Geometry: final body of the model. Coordinates: model frame, mm. A direction names the side the tool comes from. Round coordinates to 2 decimals unless told otherwise and drop trailing zeros. Order: outer loops, then holes, each group sorted by start corner. A loop starts at its lowest first (then second) coordinate and runs counter-clockwise, first axis right, second up. Notation, with made-up numbers: M 73,-15.75 L 111,-15.75 A9 ccw 111,1.25 Z; hole C -24,13 d10. An arc over 180 degrees is marked long. Return JSON: item names as keys, results as strings. Group by question number.
Q1. Cut plane B-B on x = -70. Output: boundary loops of the cut face in (y, z).
Q2. Cut plane D-D on y = 140.5. Output: boundary loops of the cut face in (x, z).
Q3. Cut plane A-A on z = 14. Count the separate pieces of the cut face and the enclosed holes in it, and give its area (3 significant figures).
Q4. Mould query, pull axis Y, two halves, no side actions, for faces 1 (the face through (20, 185, 11)), 2 (the face through (-13, 125.374, 4)), 3 (the face through (19, 132, 5)). Classes: released by +Y, released by -Y, zero draft, split by the parting line, or undercut.
Q5. Ray query, probe 1 along Y at (x, z) = (-129.5, 12); probe 2 along Y at (x, z) = (-156, 8.5); probe 3 along Y at (x, z) = (-104, 3). Return the intervals inside material, ascending.
Q6. Access query for faces 4 (the face through (3, 273.974, 3)), 5 (the face through (-50, 173, 11)), 6 (the face through (33.2, 253.5, 21.3)), 7 (the face through (-129, 156, 5)). Directions: +Z, -Z, +X, -X, +Y, -Y. A direction counts if a zero-diameter tool reaches every point of the face in a straight line with its end or side. Return the directions, or none.
Q7. Cut plane C-C on z = 27.5. Output: boundary loops of the cut face in (x, y) (3 decimals).
Q8. Contact query for flat-ended pins moving along their axis: pin 1 (13 mm diameter, centred on x = -132, y = 152, fed in from +Z); pin 2 (7.5 mm diameter, centred on x = -59.5, z = 11.5, fed in from +Y); pin 3 (4 mm diameter, centred on x = -161.5, z = 3, fed in from -Y); pin 4 (12 mm diameter, centred on x = 50.5, z = 24, fed in from +Y). Output: stop coordinate, or through.
```python
from build123d import *

# Parameters (mm, degrees)
SKETCH1_W            = 128
SKETCH1_H            = 110
SKETCH1_W_2          = 50
SKETCH1_H_2          = 70
BOSS_EXTRUDE1_DEPTH  = 5
SKETCH2_R            = 4.5
SKETCH2_R_2          = 3.025
SKETCH2_R_3          = 4.411768353
BOSS_EXTRUDE2_DEPTH  = 6
SKETCH3_W            = 194
SKETCH3_H            = 2
BOSS_EXTRUDE3_DEPTH  = 20
SKETCH6_W            = 12
SKETCH6_H            = 12
BOSS_EXTRUDE5_DEPTH  = 5
M4_CLEARANCE_HOLE1_D = 4.8
CUT_EXTRUDE1_DEPTH   = 329.83563266
FILLET2_R            = 3
FILLET3_R            = 3
SKETCH11_R           = 5
SKETCH11_R_2         = 3.025
BOSS_EXTRUDE6_DEPTH  = 30
FILLET4_R            = 3


with BuildPart() as part:
    # Sketch1 → Boss-Extrude1 (new body)
    with BuildSketch(Plane.XY):
        with Locations((-103.32475602, 215.37439567)):
            Rectangle(SKETCH1_W, SKETCH1_H)
        Polygon((26.67524398, 270.37439567), (-39.32475602, 270.37439567), (-39.32475602, 160.37439567), (-39.32475602, 125.37439567), (26.67524398, 125.37439567), (26.67524398, 195.37439567), (26.67524398, 200.37439567), align=None)
        with Locations((51.67524398, 235.37439567)):
            Rectangle(SKETCH1_W_2, SKETCH1_H_2)
    extrude(amount=BOSS_EXTRUDE1_DEPTH)

    # Sketch2 → Boss-Extrude2 (add)
    # profile 1 of 10: a face of its own
    with BuildSketch(Plane.XY.offset(5)):
        with Locations((-49.57975602, 169.52739567)):
            Circle(SKETCH2_R)
        with Locations((-49.57975602, 169.52739567)):
            Circle(SKETCH2_R_2, mode=Mode.SUBTRACT)
    # profile 2 of 10: a face of its own
    with BuildSketch(Plane.XY.offset(5)):
        with Locations((-31.18175602, 188.30539567)):
            Circle(SKETCH2_R)
        with Locations((-31.18175602, 188.30539567)):
            Circle(SKETCH2_R_2, mode=Mode.SUBTRACT)
    # profile 3 of 10: a face of its own
    with BuildSketch(Plane.XY.offset(5)):
        with Locations((-31.18175602, 131.55539567)):
            Circle(SKETCH2_R)
        with Locations((-31.18175602, 131.55539567)):
            Circle(SKETCH2_R_2, mode=Mode.SUBTRACT)
    # profile 4 of 10: a face of its own
    with BuildSketch(Plane.XY.offset(5)):
        with Locations((18.81824398, 131.55539567)):
            Circle(SKETCH2_R)
        with Locations((18.81824398, 131.55539567)):
            Circle(SKETCH2_R_2, mode=Mode.SUBTRACT)
    # profile 5 of 10: a face of its own
    with BuildSketch(Plane.XY.offset(5)):
        with Locations((18.81824398, 188.30539567)):
            Circle(SKETCH2_R)
        with Locations((18.81824398, 188.30539567)):
            Circle(SKETCH2_R_2, mode=Mode.SUBTRACT)
    # profile 6 of 10: a face of its own
    with BuildSketch(Plane.XY.offset(5)):
        with Locations((18.81824398, 261.55539567)):
            Circle(SKETCH2_R)
        with Locations((18.81824398, 261.55539567)):
            Circle(SKETCH2_R_2, mode=Mode.SUBTRACT)
    # profile 7 of 10: a face of its own
    with BuildSketch(Plane.XY.offset(5)):
        with Locations((-49.57975602, 262.49139567)):
            Circle(SKETCH2_R_3)
        with Locations((-49.57975602, 262.49139567)):
            Circle(SKETCH2_R_2, mode=Mode.SUBTRACT)
    # profile 8 of 10: a face of its own
    with BuildSketch(Plane.XY.offset(5)):
        with Locations((-154.35475602, 262.49139567)):
            Circle(SKETCH2_R)
        with Locations((-154.35475602, 262.49139567)):
            Circle(SKETCH2_R_2, mode=Mode.SUBTRACT)
    # profile 9 of 10: a face of its own
    with BuildSketch(Plane.XY.offset(5)):
        with Locations((-154.35475602, 169.52739567)):
            Circle(SKETCH2_R)
        with Locations((-154.35475602, 169.52739567)):
            Circle(SKETCH2_R_2, mode=Mode.SUBTRACT)
    # profile 10 of 10: a face of its own
    with BuildSketch(Plane.XY.offset(5)):
        with Locations((-31.18175602, 261.55539567)):
            Circle(SKETCH2_R)
        with Locations((-31.18175602, 261.55539567)):
            Circle(SKETCH2_R_2, mode=Mode.SUBTRACT)
    extrude(amount=BOSS_EXTRUDE2_DEPTH)

    # Sketch3 → Boss-Extrude3 (add)
    with BuildSketch(Plane.XY.offset(5)):
        with Locations((-70.32475602, 269.37439567)):
            Rectangle(SKETCH3_W, SKETCH3_H)
        Polygon((-167.32475602, 162.37439567), (-167.32475602, 160.37439567), (-39.32475602, 160.37439567), (-39.32475602, 125.37439567), (-37.32475602, 125.37439567), (-37.32475602, 162.37439567), align=None)
    extrude(amount=BOSS_EXTRUDE3_DEPTH)

    # Sketch6 → Boss-Extrude5 (add)
    with BuildSketch(Plane(origin=(0, 0, 0), x_dir=(-1, 0, 0), z_dir=(0, 0, -1))):
        with Locations((131.32475602, 154.37439567)):
            Rectangle(SKETCH6_W, SKETCH6_H)
        with Locations((159.32475602, 276.37439567)):
            Rectangle(SKETCH6_W, SKETCH6_H)
        with Locations((45.32475602, 154.37439567)):
            Rectangle(SKETCH6_W, SKETCH6_H)
        with Locations((-5.67524398, 276.37439567)):
            Rectangle(SKETCH6_W, SKETCH6_H)
    extrude(amount=-BOSS_EXTRUDE5_DEPTH)

    # M4 Clearance Hole1 (through all)
    with Locations(Plane.XY.offset(5)):
        with Locations((-131.32475602, 154.37439567), (-159.32475602, 276.37439567), (5.67524398, 276.37439567), (-45.32475602, 154.37439567)):
            Hole(M4_CLEARANCE_HOLE1_D / 2)

    # Sketch10 → Cut-Extrude1 (cut, through all)
    with BuildSketch(Plane.XY.offset(5)):
        with BuildLine():
            ThreePointArc((-131.32475602, 151.97439567), (-133.72475602, 154.37439567), (-131.32475602, 156.77439567))
            Line((-131.32475602, 156.77439567), (-137.32475602, 156.77439567))
            Line((-137.32475602, 156.77439567), (-137.32475602, 151.97439567))
            Line((-137.32475602, 151.97439567), (-131.32475602, 151.97439567))
        make_face()
        with BuildLine():
            ThreePointArc((-159.32475602, 273.97439567), (-161.72475602, 276.37439567), (-159.32475602, 278.77439567))
            Line((-159.32475602, 278.77439567), (-165.32475602, 278.77439567))
            Line((-165.32475602, 278.77439567), (-165.32475602, 273.97439567))
            Line((-165.32475602, 273.97439567), (-159.32475602, 273.97439567))
        make_face()
        with BuildLine():
            ThreePointArc((5.67524398, 273.97439567), (3.27524398, 276.37439567), (5.67524398, 278.77439567))
            Line((5.67524398, 278.77439567), (-0.32475602, 278.77439567))
            Line((-0.32475602, 278.77439567), (-0.32475602, 273.97439567))
            Line((-0.32475602, 273.97439567), (5.67524398, 273.97439567))
        make_face()
        with BuildLine():
            ThreePointArc((-45.32475602, 151.97439567), (-47.72475602, 154.37439567), (-45.32475602, 156.77439567))
            Line((-45.32475602, 156.77439567), (-51.32475602, 156.77439567))
            Line((-51.32475602, 156.77439567), (-51.32475602, 151.97439567))
            Line((-51.32475602, 151.97439567), (-45.32475602, 151.97439567))
        make_face()
    extrude(amount=-CUT_EXTRUDE1_DEPTH, mode=Mode.SUBTRACT)

    # Fillet2
    # the kernel refuses this fillet: 3 mm, written as the material it adds along each edge
    with BuildSketch(Plane(origin=(-137.32475602, 160.37439567, 0), x_dir=(-1, 0, 0), z_dir=(0, 0, 1)), Plane(origin=(-153.32475602, 270.37439567, 0), x_dir=(1, 0, 0), z_dir=(0, 0, 1)), Plane(origin=(-51.32475602, 160.37439567, 0), x_dir=(-1, 0, 0), z_dir=(0, 0, 1)), Plane(origin=(11.67524398, 270.37439567, 0), x_dir=(1, 0, 0), z_dir=(0, 0, 1))) as fillet2_piece_1:
        with BuildLine():
            CenterArc((FILLET2_R, FILLET2_R), FILLET2_R, 180, 90)
            Line((0, FILLET2_R), (0, 0))
            Line((0, 0), (FILLET2_R, 0))
        make_face()
    extrude(amount=5)
    with BuildSketch(Plane(origin=(-125.32475602, 160.37439567, 0), x_dir=(1, 0, 0), z_dir=(0, 0, 1)), Plane(origin=(-39.32475602, 148.37439567, 0), x_dir=(0, -1, 0), z_dir=(0, 0, 1)), Plane(origin=(-0.32475602, 270.37439567, 0), x_dir=(-1, 0, 0), z_dir=(0, 0, 1))) as fillet2_piece_2:
        with BuildLine():
            CenterArc((FILLET2_R, -FILLET2_R), FILLET2_R, 90, 90)
            Line((0, -FILLET2_R), (0, 0))
            Line((0, 0), (FILLET2_R, 0))
        make_face()
    extrude(amount=5)
    with BuildSketch(Plane(origin=(-165.32475602, 270.37439567, 0), x_dir=(-1, 0, 0), z_dir=(0, 0, 1))) as fillet2_piece_3:
        with BuildLine():
            CenterArc((3, -2.828427125), FILLET2_R, 109.471220634, 70.528779366)
            Line((0, -2.828427125), (0, 0))
            Line((0, 0), (2, 0))
        make_face()
    extrude(amount=5)
    # the kernel refuses this fillet: 3 mm, written as the material it takes off along each edge
    with BuildSketch(Plane(origin=(-125.32475602, 148.37439567, -7.5), x_dir=(0, 1, 0), z_dir=(0, 0, 1))) as fillet2_2_piece_1:
        with BuildLine():
            CenterArc((FILLET2_R, FILLET2_R), FILLET2_R, 180, 90)
            Line((0, FILLET2_R), (0, 0))
            Line((0, 0), (FILLET2_R, 0))
        make_face()
    extrude(amount=20, mode=Mode.SUBTRACT)
    with BuildSketch(Plane(origin=(-153.32475602, 282.37439567, -7.5), x_dir=(0, -1, 0), z_dir=(0, 0, 1)), Plane(origin=(11.67524398, 282.37439567, -7.5), x_dir=(0, -1, 0), z_dir=(0, 0, 1))) as fillet2_2_piece_2:
        with BuildLine():
            CenterArc((FILLET2_R, -FILLET2_R), FILLET2_R, 90, 90)
            Line((0, -FILLET2_R), (0, 0))
            Line((0, 0), (FILLET2_R, 0))
        make_face()
    extrude(amount=20, mode=Mode.SUBTRACT)

    # Fillet3
    fillet3_edges = [part.edges().sort_by_distance(p)[0] for p in [
        (76.67524398, 270.37439567, 2.5),
        (76.67524398, 200.37439567, 2.5),
        (26.67524398, 200.37439567, 2.5),
        (26.67524398, 125.37439567, 2.5),
        (-39.32475602, 160.37439567, 15),
    ]]
    fillet(fillet3_edges, radius=FILLET3_R)

    # Sketch11 → Boss-Extrude6 (add)
    # profile 1 of 4: a face of its own
    with BuildSketch(Plane.XY.offset(5)):
        with Locations((34.31824398, 258.37439567)):
            Circle(SKETCH11_R)
        with Locations((34.31824398, 258.37439567)):
            Circle(SKETCH11_R_2, mode=Mode.SUBTRACT)
    # profile 2 of 4: a face of its own
    with BuildSketch(Plane.XY.offset(5)):
        with Locations((64.31824398, 258.37439567)):
            Circle(SKETCH11_R)
        with Locations((64.31824398, 258.37439567)):
            Circle(SKETCH11_R_2, mode=Mode.SUBTRACT)
    # profile 3 of 4: a face of its own
    with BuildSketch(Plane.XY.offset(5)):
        with Locations((64.31824398, 212.37439567)):
            Circle(SKETCH11_R)
        with Locations((64.31824398, 212.37439567)):
            Circle(SKETCH11_R_2, mode=Mode.SUBTRACT)
    # profile 4 of 4: a face of its own
    with BuildSketch(Plane.XY.offset(5)):
        with Locations((34.31824398, 212.37439567)):
            Circle(SKETCH11_R)
        with Locations((34.31824398, 212.37439567)):
            Circle(SKETCH11_R_2, mode=Mode.SUBTRACT)
    extrude(amount=BOSS_EXTRUDE6_DEPTH)

    # Fillet4
    fillet4_edges = [part.edges().sort_by_distance(p)[0] for p in [
        (29.31824398, 258.37439567, 5),
        (59.31824398, 258.37439567, 5),
        (59.31824398, 212.37439567, 5),
        (29.31824398, 212.37439567, 5),
    ]]
    fillet(fillet4_edges, radius=FILLET4_R)


solid = part.part
```
Result sheet:
{
 "1": {"outline": "M 160.37,0 L 270.37,0 L 270.37,25 L 268.37,25 L 268.37,5 L 162.37,5 L 162.37,25 L 160.37,25 Z"},
 "2": {"outline": "M -39.32,0 L 26.68,0 L 26.68,5 L -37.32,5 L -37.32,25 L -39.32,25 Z"},
 "3": {"separate pieces": "6", "enclosed holes": "4", "area": "919 mm²"},
 "4": {"face 1": "zero draft", "face 2": "released by -Y", "face 3": "undercut"},
 "5": {"probe 1": "y = 160.37 to 162.37, 268.37 to 270.37", "probe 2": "y = 160.37 to 162.37, 165.34 to 166.99, 172.07 to 173.72, 258.3 to 259.95, 265.03 to 266.68, 268.37 to 270.37", "probe 3": "y = 160.37 to 270.37"},
 "6": {"face 4": "+Z, -Z", "face 5": "+Z, +X, -X", "face 6": "+Z", "face 7": "+Z, -X, -Y"},
 "7": {"outline": "C 34.318,212.374 d10; C 34.318,258.374 d10; C 64.318,212.374 d10; C 64.318,258.374 d10; hole C 34.318,212.374 d6.05; hole C 34.318,258.374 d6.05; hole C 64.318,212.374 d6.05; hole C 64.318,258.374 d6.05"},
 "8": {"pin 1": "stops at z = 5", "pin 2": "stops at y = 270.37", "pin 3": "stops at y = 160.37", "pin 4": "passes through"}
}
